Model file for the job. Use its own axes, mm. A direction names the side the tool comes from. Round coordinates to 2 decimals unless told otherwise and drop trailing zeros. Order: outer loops, then holes, each group sorted by start corner. A loop starts at its lowest first (then second) coordinate and runs counter-clockwise, first axis right, second up. Notation, with made-up numbers: (-3.75, 31) - (37.25, 31) arc R13 cw to (37.25, 43) - close; hole circle Ø8 at (-10.5, -5). An arc over 180 degrees is marked (long way). Answer as CSV lines item,"result". Start each with the question number.
1. Pin check, flat tips, straight feed: pin 1 Ø5.5 at (x, y) = (-5.5, 73) entering from +Z; pin 2 Ø1 at (x, y) = (14.5, 55.5) entering from +Z; pin 3 Ø12 at (x, z) = (-14.5, 44) entering from -Y. Stop position of each tip, or through.
2. Pull direction X, two halves, no side cores. Call faces 5 (the face through (0, 73, 127)), 6 (the face through (-71.917, 11.956, 139.878)), 7 (the face through (50, 50, 152.4)): released by +X, released by -X, zero draft, split by the parting line, or undercut.
3. Band-saw the part on B-B on z = 37.5. List the corners of the cut face in (x, y).
4. Wall check: line 1 along X through (y, z) = (0, 95); line 2 along Z through (x, y) = (-14, 24). Give the ranges that are in metal, low to high. Write a range as [from, to].
5. Band-saw the part on A-A on y = 0. List the corners of the cut face in (x, z), then the cut area to 3 significant figures.
6. 3-axis set-ups, long thin cutter, end or side, ignore diameter. For faces 1 (the face through (-11.956, -71.917, 139.878)), 2 (the face through (-1, 1, 6.35)), 3 (the face through (-11.986, 72.003, 139.878)), 4 (the face through (-73, 0, 127)): which of +Z, -Z, +X, -X, +Y, -Y reach the whole face in a straight line?
```python
from build123d import *

# Parameters (mm, degrees)
F0_R     = 76.2
F1_DEPTH = 152.4
F2_R     = 12.7
F3_T     = -6.35
F4_R     = 12.7
F5_DEPTH = 25.4


with BuildPart() as f1:
    # F0 (on Top) → F1 (new body)
    with BuildSketch(Plane.XY):
        Circle(F0_R)
    extrude(amount=F1_DEPTH)

    # F2
    f2_edges = [f1.edges().sort_by_distance(p)[0] for p in [
        (-76.2, 0, 0),
    ]]
    fillet(f2_edges, radius=F2_R)

    # F3
    f3_openings = [f1.faces().sort_by_distance(p)[0] for p in [
        (0, 0, 152.4),
    ]]
    offset(amount=F3_T, openings=f3_openings)

    # F4 (on face) → F5 (cut)
    with BuildSketch(Plane.XY.offset(152.4)):
        with Locations((0, 76.2)):
            Circle(F4_R)
        with Locations((-76.2, 0)):
            Circle(F4_R)
        with Locations((0, -76.2)):
            Circle(F4_R)
        with Locations((76.2, 0)):
            Circle(F4_R)
    extrude(amount=-F5_DEPTH, mode=Mode.SUBTRACT)


solid = f1.part
```
Reply:
1,pin 1,"stops at z = 127"
1,pin 2,"stops at z = 6.35"
1,pin 3,"stops at y = -75.72"
2,face 5,"undercut"
2,face 6,"released by -X"
2,face 7,"zero draft"
3,outline,"circle Ø152.4 at (0, 0); hole circle Ø139.7 at (0, 0)"
4,line 1,"x = [-76.2, -69.85], [69.85, 76.2]"
4,line 2,"z = [0, 6.35]"
5,outline,"(-76.2, 12.7) arc R12.7 ccw to (-63.5, 0) - (63.5, 0) arc R12.7 ccw to (76.2, 12.7) - (76.2, 127) - (69.85, 127) - (69.85, 12.7) arc R6.35 cw to (63.5, 6.35) - (-63.5, 6.35) arc R6.35 cw to (-69.85, 12.7) - (-69.85, 127) - (-76.2, 127) - close"
5,area,"2,450 mm2"
6,face 1,"+Z, -Y"
6,face 2,"+Z"
6,face 3,"+Z, +Y"
6,face 4,"+Z, -X"
